Autodesk Inventor part; units mm, degrees
ref_plane "YZ Plane" through (0, 0, 0) normal (1, 0, 0) x (0, 1, 0)
ref_plane "XZ Plane" through (0, 0, 0) normal (0, 1, 0) x (-1, 0, 0)
ref_plane "XY Plane" through (0, 0, 0) normal (0, 0, 1) x (1, 0, 0)
sketch "Boceto1" plane through (0, 0, 0) normal (1, 0, 0) x (0, 1, 0)
  line L0 (-6.321, 6.321) -> (6.321, 6.321) construction
  line L1 (6.321, 6.321) -> (6.321, -6.321) construction
  line L2 (6.321, -6.321) -> (-6.321, -6.321) construction
  line L3 (-6.321, -6.321) -> (-6.321, 6.321) construction
  line L4 (-6.321, 6.321) -> (6.321, -6.321) construction
  line L5 (6.321, 6.321) -> (-6.321, -6.321) construction
  circle A0 centre (6.321, -6.321) radius 0.875
  line L6 (0, 0) -> (7.9878, 0) construction
  circle A1 centre (6.321, 6.321) radius 0.875
  line L7 (0, 0) -> (0, -13.4562) construction
  circle A2 centre (-6.321, -6.321) radius 0.875
  circle A3 centre (-6.321, 6.321) radius 0.875
  circle A4 centre (0, 0) radius 5.5
  line L8 (10, 20) -> (-20, 20)
  line L9 (-20, 20) -> (-20, -20)
  line L10 (-20, -20) -> (10, -20)
  line L11 (10, -20) -> (10, 20)
  dimension "d0" = 12.642
  dimension "d1" = 12.642
  dimension "d2" = 1.75
  dimension "d3" = 11
  dimension "d4" = 30
  dimension "d6" = 20
  dimension "d7" = 10
  dimension "d26" = 20
extrude "Extrusión1" add sketch "Boceto1" along normal blind 2
sketch "Boceto2" plane through (0, -20, -20) normal (0, -1, 0) x (1, 0, 0)
  line L0 (2, 0) -> (2, 40)
  line L1 (2, 40) -> (-38, 40)
  line L2 (-38, 40) -> (-38, 0)
  line L3 (-38, 0) -> (2, 0)
  line L4 (2, 0) -> (2, 40)
  point P0 (0, 20)
  point P1 (2, 0)
  dimension "d10" = 40
  dimension "d11" = 40
extrude "Extrusión2" add sketch "Boceto2" along normal blind 2
fillet "Empalme1" radius 1.5 1 edges at (0, -20, 0)
fillet "Empalme2" radius 1 5 edges at (1, 10, 20) (1, 10, -20) (-38, -21, 20) (-38, -21, -20) (2, -22, 0)
sketch "Boceto4" plane through (0, -20, -20) normal (0, 1, 0) x (1, 0, 0)
  circle A0 centre (-13, -10) radius 2.5
  circle A1 centre (-13, -30) radius 2.5
  circle A2 centre (-28, -10) radius 2.5
  circle A3 centre (-28, -30) radius 2.5
  line L0 (-1.5, -40) -> (-37, -40)
  line L1 (-38, -39) -> (-38, -1)
  point P0 (0, -20)
  dimension "d27" = 5
  dimension "d28" = 5
  dimension "d29" = 5
  dimension "d30" = 5
  dimension "d31" = 10
  dimension "d32" = 20
  dimension "d33" = 20
  dimension "d34" = 15
  dimension "d35" = 10
extrude "Extrusión4" cut sketch "Boceto4" against normal through all
sketch "Boceto5" plane through (2, 0, 0) normal (1, 0, 0) x (0, 0, -1)
  line L0 (20, -21) -> (-20, -21)
  line L1 (20, 9) -> (20, -21)
  arc A0 (20, 9) -> (19, 10) centre (19, 9) ccw
  line L2 (19, 10) -> (-19, 10)
  arc A1 (-19, 10) -> (-20, 9) centre (-19, 9) ccw
  line L3 (-20, 9) -> (-20, -21)
  circle A2 centre (0, 0) radius 5.5
  circle A3 centre (-6.321, -6.321) radius 0.875
  circle A4 centre (6.321, -6.321) radius 0.875
  circle A5 centre (-6.321, 6.321) radius 0.875
  circle A6 centre (6.321, 6.321) radius 0.875
extrude "Extrusión5" add sketch "Boceto5" against normal blind 2 contours A2 | A3 | A4 | A5 | A6
sketch "Boceto7" plane through (0, 0, 0) normal (-1, 0, 0) x (0, 0, 1)
  arc A0 (-19, 10) -> (-20, 9) centre (-19, 9) ccw
  line L0 (-20, -18.5) -> (-20, 9)
  line L1 (20, -18.5) -> (-20, -18.5)
  line L2 (20, 9) -> (20, -18.5)
  arc A1 (20, 9) -> (19, 10) centre (19, 9) ccw
  line L3 (-19, 10) -> (19, 10)
  line L4 (-20, -18.5) -> (20, -18.5)
  line L5 (20, -18.5) -> (20, 31.5)
  line L6 (20, 31.5) -> (-20, 31.5)
  line L7 (-20, 31.5) -> (-20, -18.5)
  point P0 (0, 0)
  dimension "d42" = 40
  dimension "d43" = 50
extrude "Extrusión7" add sketch "Boceto7" against normal blind 2 contours A0 L7 L6 L5 A1 L3
fillet "Empalme3" radius 2 2 edges at (1, 31.5, -20) (1, 31.5, 20)
sketch "Boceto8" plane through (0, 0, 0) normal (-1, 0, 0) x (0, 0, 1)
  line L0 (-18, 31.5) -> (18, 31.5) construction
  line L1 (0, 31.5) -> (0, 13.8) construction
  line L2 (-20, -18.5) -> (-20, 29.5) construction
  line L3 (-20, 13.8) -> (19.9852, 13.8) construction
  line L4 (-20, 13.8) -> (-7.75, 13.8) construction
  circle A0 centre (-7.75, 13.8) radius 1.5
  circle A1 centre (5.25, 13.8) radius 1.5
  point P0 (0, 0)
  dimension "d47" = 17.7
  dimension "d48" = 12.25
  dimension "d49" = 3
  dimension "d50" = 3
  dimension "d51" = 13
extrude "Extrusión8" cut sketch "Boceto8" against normal blind 2
sketch "Boceto9" plane through (0, 0, 0) normal (-1, 0, 0) x (0, 0, 1)
  line L0 (-10, 23.5) -> (9, 23.5)
  line L1 (18, 31.5) -> (-18, 31.5)
  line L2 (9, 23.5) -> (-10, 23.5) construction
  line L3 (9, 25.5) -> (-10, 25.5)
  line L4 (-10, 21.5) -> (9, 21.5)
  arc A0 (9, 21.5) -> (9, 25.5) centre (9, 23.5) ccw
  arc A1 (-10, 25.5) -> (-10, 21.5) centre (-10, 23.5) ccw
  line L5 (-20, -18.5) -> (-20, 29.5)
  point P0 (0, 0)
  point P1 (0, 31.5)
  point P2 (0, 31.5)
  point P3 (-0.5, 23.5)
  dimension "d56" = 8
  dimension "d57" = 9
  dimension "d58" = 10
  dimension "d59" = 4
extrude "Extrusión9" cut sketch "Boceto9" against normal blind 2
sketch "Boceto11" plane through (0, 0, 0) normal (-1, 0, 0) x (0, 0, 1)
  circle A0 centre (0, 0) radius 5.5
  circle A1 centre (5.25, 13.8) radius 1.5
  dimension "d64" = 13.8
sketch "Boceto3" plane through (0, -20, -20) normal (0, 1, 0) x (1, 0, 0)
  line L0 (0, -40) -> (0, 0)
  line L1 (-28, 0) -> (0, 0)
  line L2 (-28, -40) -> (-28, 0)
  line L3 (0, -40) -> (-28, -40)
  line L4 (-6.125, -3.125) -> (-6.125, -36.875) construction
  line L5 (-7.25, -3.125) -> (-7.25, -36.875)
  line L6 (-5, -36.875) -> (-5, -3.125)
  arc A0 (-5, -3.125) -> (-7.25, -3.125) centre (-6.125, -3.125) ccw
  arc A1 (-7.25, -36.875) -> (-5, -36.875) centre (-6.125, -36.875) ccw
  line L7 (-21.875, -3.125) -> (-21.875, -36.875) construction
  line L8 (-23, -3.125) -> (-23, -36.875)
  line L9 (-20.75, -36.875) -> (-20.75, -3.125)
  arc A2 (-20.75, -3.125) -> (-23, -3.125) centre (-21.875, -3.125) ccw
  arc A3 (-23, -36.875) -> (-20.75, -36.875) centre (-21.875, -36.875) ccw
  point P0 (0, -20)
  point P1 (-6.125, -20)
  point P2 (-21.875, -20)
  point P3 (-21.875, -38)
  point P4 (-21.875, -2)
  point P5 (-6.125, -38)
  point P6 (-6.125, -2)
  dimension "d14" = 2.25
  dimension "d15" = 2.25
  dimension "d16" = 5
  dimension "d17" = 2
  dimension "d18" = 2
  dimension "d19" = 2
  dimension "d20" = 2
  dimension "d21" = 5
equation "\"Radio_pliegue\" = Grosor"
equation "\"Anchura_desahogo_plegado\" = Grosor"
equation "\"Profundidad_desahogo_plegado\" = 0.5 * Grosor"
equation "\"Tamaño_destalonado\" = 4 * Grosor"
equation "\"Remanente_mínimo\" = 2 * Grosor"
equation "\"Radiodetransición\" = Radio_pliegue"
equation "\"Tamaño_de_radio_de_Jacobi\" = Radio_pliegue"
equation "\"TamañoSeparación\" = Grosor"
properties part number "BRACKET_SENSOR" material "Aluminio 6061"
Read the model definition and answer for the solid it produces. Units are mm, in the model's axes. A direction names the side the tool comes from. Coordinates: 2 decimals unless noted, no trailing zeros. Loops run counter-clockwise (first coordinate to the right, second up) from the corner with the lowest first, then second, coordinate; pieces in that order, holes last. Notation, with made-up numbers: (-18.75, 20.25) - (23.25, 20.25) arc R29 ccw to (23.25, 58.25) - close; hole circle Ø7 at (76, 23). An arc over 180 degrees is marked (long way). Answer in a Markdown table with one row per item.
1. Which of the six approach directions +Z, -Z, +X, -X, +Y, -Y give full straight-line access (tool end or side, diameter ignored) to faces 5 (the face through (1, 21.5, -1)), 6 (the face through (-19, -22, 0)), 7 (the face through (-20, -20, 0))?
Conclusion:
| item | result |
|---|---|
| face 5 | +X, -X |
| face 6 | +Z, -Z, +X, -X, -Y |
| face 7 | +Z, -Z, -X, +Y |
2. Find section D-D, the plane z = -16.5. Write down the section's boundary in (x, y), then the cut area to 3 significant figures.
Conclusion:
| item | result |
|---|---|
| outline | (-38, -22) - (1, -22) arc R1 ccw to (2, -21) - (2, 31.5) - (0, 31.5) - (0, -18.5) arc R1.5 cw to (-1.5, -20) - (-38, -20) - close |
| area | 183 mm² |
3. Determine the mould class of faces 1 (the face through (1, 31.5, 0)), 2 (the face through (1.01, 30.9, -19.43)), 3 (the face through (-28.54, -20.99, 12.44)), 4 (the face through (0.986, 12.336, -8.075)) for opening direction Z: +Z half, -Z half, draft (parallel to the pull), parting line (faces both ways), or undercut.
Conclusion:
| item | result |
|---|---|
| face 1 | draft |
| face 2 | -Z half |
| face 3 | undercut |
| face 4 | undercut |
4. Find section C-C, the plane z = 1. Write down the section's boundary in (x, y).
Conclusion:
| item | result |
|---|---|
| outline | (-38, -22) - (1, -22) arc R1 ccw to (2, -21) - (2, 21.5) - (0, 21.5) - (0, -18.5) arc R1.5 cw to (-1.5, -20) - (-38, -20) - close; (0, 25.5) - (2, 25.5) - (2, 31.5) - (0, 31.5) - close |
5. Straight lines are drawn through the part: line 1 (X direction, y = -20.7, z = -10); line 2 (Z direction, x = -28, y = -20.9); line 3 (Y direction, x = 0.7, z = 5.25). For each, find the intervals that lie inside material, in ascending order.
Conclusion:
| item | result |
|---|---|
| line 1 | x = -38 to -30.5, -25.5 to -15.5, -10.5 to 2 |
| line 2 | z = -20 to -12.5, -7.5 to 7.5, 12.5 to 20 |
| line 3 | y = -22 to 12.3, 15.3 to 21.5, 25.5 to 31.5 |
6. Given pin 1 (1 mm diameter, centred on y = 11, z = 13, fed in from -X); pin 2 (4 mm diameter, centred on x = -13, z = -10, fed in from +Y); pin 3 (11 mm diameter, centred on x = -18.5, z = 2.5, fed in from +Y), each flat-ended and moving along its own axis, determine where each tip first touches the part or whether it passes through.
Conclusion:
| item | result |
|---|---|
| pin 1 | stops at x = 0 |
| pin 2 | passes through |
| pin 3 | stops at y = -20 |
7. Find section A-A, the plane z = 5.25. Write down the section's boundary in (x, y).
Conclusion:
| item | result |
|---|---|
| outline | (-38, -22) - (1, -22) arc R1 ccw to (2, -21) - (2, 12.3) - (0, 12.3) - (0, -18.5) arc R1.5 cw to (-1.5, -20) - (-38, -20) - close; (0, 15.3) - (2, 15.3) - (2, 21.5) - (0, 21.5) - close; (0, 25.5) - (2, 25.5) - (2, 31.5) - (0, 31.5) - close |
8. Find section B-B, the plane y = 23.5. Write down the section's boundary in (x, z).
Conclusion:
| item | result |
|---|---|
| outline | (0, -20) - (2, -20) - (2, -12) - (0, -12) - close; (0, 11) - (2, 11) - (2, 20) - (0, 20) - close |
